Here's how the part is built. I have some questions about the finished solid (model axes, mm). Face numbers are marked on the shaded views. A direction names the side the tool comes from. Coordinates: 2 decimals unless noted, no trailing zeros. Loops run counter-clockwise (first coordinate to the right, second up) from the corner with the lowest first, then second, coordinate; pieces in that order, holes last. Notation, with made-up numbers: M 55.5,50.25 L 82.5,50.25 A25 ccw 82.5,64.25 Z; hole C 35.25,42.5 d2. An arc over 180 degrees is marked long. Use CSV: the item, a comma, the result in double quotes. Start each with the question number.
Q1. If we section it at B-B (z = 23): Please give me the cut outline in (x, y) (3 decimals).
Q2. If we section it at C-C (x = 12): Please give me the cut outline in (y, z) (3 decimals).
Q3. For pin 1 Ø8.5 at (y, z) = (10.5, -6.5) entering from +X (3 decimals); pin 2 Ø12 at (x, y) = (19.5, 17) entering from +Z; pin 3 Ø5.5 at (y, z) = (13.5, 12) entering from -X (3 decimals); pin 4 Ø1.5 at (x, y) = (30.5, 11.5) entering from -Z (3 decimals), each with a flat end and sliding along its axis, tell me the tip position at first contact or that it passes through.
Q4. Which directions (+Z, -Z, +X, -X, +Y, -Y) give clear straight access to the entire face, cutting with the end or side of a thin tool? Please do the marked faces 1, 2 and 3.
Q5. If we section it at D-D (z = -3): Please give me the cut outline in (x, y) (3 decimals), and give its area (3 significant figures).
Q6. Please list where these lines run through material, in increasing order: probe 1 along Z at (x, y) = (33.5, 10.16) (3 decimals); probe 2 along X at (y, z) = (14.75, 19) (3 decimals); probe 3 along X at (y, z) = (20, 4). Write a range as [from, to].
Q7. If we mould it in two halves opening along Z, with no side actions, what happens to the marked faces 4, 5 and 6? For each: +Z half, -Z half, draft (parallel to the pull), parting line (faces both ways), or undercut.
Q8. If we section it at A-A (y = 10.16): Please give me the cut outline in (x, z) (3 decimals), and give its area (3 significant figures).
from build123d import *

# Parameters (mm, degrees)
SKETCH1_W           = 82.55
SKETCH1_H           = 82.55
BOSS_EXTRUDE1_DEPTH = 19.05
BOSS_EXTRUDE2_START = 19.05
SKETCH1_3_W         = 88.9
SKETCH1_3_H         = 88.9
SKETCH1_3_W_2       = 82.55
SKETCH1_3_H_2       = 82.55
BOSS_EXTRUDE2_DEPTH = 9.525
FILLET1_R           = 6.35
CHAMFER1_SIZE       = 6.35
SKETCH2_R           = 4
CUT_EXTRUDE2_DEPTH  = 101.703072197


with BuildPart() as part:
    # Sketch1 → Boss-Extrude1 (new body)
    with BuildSketch(Plane(origin=(0, 0, 0), x_dir=(1, 0, 0), z_dir=(0, 1, 0))):
        Rectangle(SKETCH1_W, SKETCH1_H)
        with BuildLine():
            ThreePointArc((-27.5336, 31.75), (-30.515045032, 30.515045032), (-31.75, 27.5336))
            Line((-31.75, 27.5336), (-31.75, -27.5336))
            ThreePointArc((-31.75, -27.5336), (-30.515045032, -30.515045032), (-27.5336, -31.75))
            Line((-27.5336, -31.75), (27.5336, -31.75))
            ThreePointArc((27.5336, -31.75), (30.515045032, -30.515045032), (31.75, -27.5336))
            Line((31.75, -27.5336), (31.75, 27.5336))
            ThreePointArc((31.75, 27.5336), (30.515045032, 30.515045032), (27.5336, 31.75))
            Line((27.5336, 31.75), (-27.5336, 31.75))
        make_face(mode=Mode.SUBTRACT)
    extrude(amount=BOSS_EXTRUDE1_DEPTH)

    # Sketch1<3> → Boss-Extrude2 (add)
    # profile 1 of 2: a face of its own
    with BuildSketch(Plane(origin=(0, 0, 0), x_dir=(1, 0, 0), z_dir=(0, 1, 0)).offset(BOSS_EXTRUDE2_START)):
        Rectangle(SKETCH1_3_W, SKETCH1_3_H)
        Rectangle(SKETCH1_3_W_2, SKETCH1_3_H_2, mode=Mode.SUBTRACT)
    # profile 2 of 2: a face of its own
    with BuildSketch(Plane(origin=(0, 0, 0), x_dir=(1, 0, 0), z_dir=(0, 1, 0)).offset(BOSS_EXTRUDE2_START)):
        Rectangle(SKETCH1_3_W_2, SKETCH1_3_H_2)
        with BuildLine():
            ThreePointArc((-27.5336, 31.75), (-30.515045032, 30.515045032), (-31.75, 27.5336))
            Line((-31.75, 27.5336), (-31.75, -27.5336))
            ThreePointArc((-31.75, -27.5336), (-30.515045032, -30.515045032), (-27.5336, -31.75))
            Line((-27.5336, -31.75), (27.5336, -31.75))
            ThreePointArc((27.5336, -31.75), (30.515045032, -30.515045032), (31.75, -27.5336))
            Line((31.75, -27.5336), (31.75, 27.5336))
            ThreePointArc((31.75, 27.5336), (30.515045032, 30.515045032), (27.5336, 31.75))
            Line((27.5336, 31.75), (-27.5336, 31.75))
        make_face(mode=Mode.SUBTRACT)
    extrude(amount=BOSS_EXTRUDE2_DEPTH)

    # Fillet1
    fillet1_edges = [part.edges().sort_by_distance(p)[0] for p in [
        (41.275, 9.525, -41.275),
        (41.275, 9.525, 41.275),
        (-41.275, 9.525, 41.275),
        (-41.275, 9.525, -41.275),
    ]]
    fillet(fillet1_edges, radius=FILLET1_R)

    # Chamfer1
    chamfer1_edges = [part.edges().sort_by_distance(p)[0] for p in [
        (44.45, 28.575, 0),
        (0, 28.575, 44.45),
        (0, 28.575, -44.45),
        (-44.45, 28.575, 0),
    ]]
    chamfer(chamfer1_edges, length=CHAMFER1_SIZE)

    # Sketch2 → Cut-Extrude2 (cut, through all)
    with BuildSketch(Plane.ZY.offset(41.275)):
        with Locations(Location((-25.4, 10.16, 0), (0, 0, 237.764531712))):
            Circle(SKETCH2_R)
        with Locations(Location((25.4, 10.16, 0), (0, 0, 57.764531712))):
            Circle(SKETCH2_R)
    extrude(amount=-CUT_EXTRUDE2_DEPTH, mode=Mode.SUBTRACT)


solid = part.part
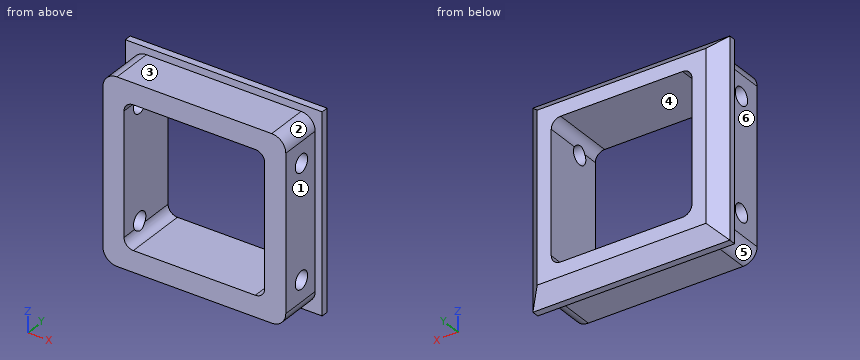
Results below:
1,outline,"M -44.45,19.05 L -41.275,19.05 L -41.275,13.36 L -31.75,13.36 L -31.75,28.575 L -38.1,28.575 L -44.45,22.225 Z; M -41.275,0 L -31.75,0 L -31.75,6.96 L -41.275,6.96 Z; M 31.75,0 L 41.275,0 L 41.275,6.96 L 31.75,6.96 Z; M 31.75,13.36 L 41.275,13.36 L 41.275,19.05 L 44.45,19.05 L 44.45,22.225 L 38.1,28.575 L 31.75,28.575 Z"
2,outline,"M 0,-41.275 L 19.05,-41.275 L 19.05,-44.45 L 22.225,-44.45 L 28.575,-38.1 L 28.575,-31.75 L 0,-31.75 Z; M 0,31.75 L 28.575,31.75 L 28.575,38.1 L 22.225,44.45 L 19.05,44.45 L 19.05,41.275 L 0,41.275 Z"
3,pin 1,"x = 41.275"
3,pin 2,"z = 44.45"
3,pin 3,"x = -41.275"
3,pin 4,"z = -41.275"
4,face 1,"+Z, -Z, +X, -Y"
4,face 2,"+Z, +X, -Y"
4,face 3,"+Z, +X, -X, -Y"
5,outline,"M -44.45,19.05 L -41.275,19.05 L -41.275,0 L -31.75,0 L -31.75,28.575 L -38.1,28.575 L -44.45,22.225 Z; M 31.75,0 L 41.275,0 L 41.275,19.05 L 44.45,19.05 L 44.45,22.225 L 38.1,28.575 L 31.75,28.575 Z"
5,area,"565 mm^2"
6,probe 1,"[-41.275, -29.4], [-21.4, 21.4], [29.4, 41.275]"
6,probe 2,"[-41.275, -31.75], [31.75, 41.275]"
6,probe 3,"[-44.45, -31.75], [31.75, 44.45]"
7,face 4,"undercut"
7,face 5,"-Z half"
7,face 6,"draft"
8,outline,"M -41.275,-34.925 A6.35 ccw -34.925,-41.275 L 34.925,-41.275 A6.35 ccw 41.275,-34.925 L 41.275,-29.4 L 31.314,-29.4 A4.216 cw 27.534,-31.75 L -27.534,-31.75 A4.216 cw -31.314,-29.4 L -41.275,-29.4 Z; M -41.275,-21.4 L -31.75,-21.4 L -31.75,21.4 L -41.275,21.4 Z; M -41.275,29.4 L -31.314,29.4 A4.216 cw -27.534,31.75 L 27.534,31.75 A4.216 cw 31.314,29.4 L 41.275,29.4 L 41.275,34.925 A6.35 ccw 34.925,41.275 L -34.925,41.275 A6.35 ccw -41.275,34.925 Z; M 31.75,-21.4 L 41.275,-21.4 L 41.275,21.4 L 31.75,21.4 Z"
8,area,"2,460 mm^2"
